Design review of the part built by this model. Coordinates are the model's own, in mm. A direction names the side the tool comes from. Coordinates: 2 decimals unless noted, no trailing zeros. Loops run counter-clockwise (first coordinate to the right, second up) from the corner with the lowest first, then second, coordinate; pieces in that order, holes last. Notation, with made-up numbers: (42.25, -35) -> (66.25, -35) arc R21 cw to (66.25, 4) -> close; hole circle Ø9 at (43.5, -30). An arc over 180 degrees is marked (long way). Answer in a Markdown table with one row per item.
```python
from build123d import *

# Parameters (mm, degrees)
F0_R     = 50.8
F1_DEPTH = 76.2
F2_DEPTH = 381
F3_R     = 25.4


with BuildPart() as f1:
    # F0 (on Front) → F1 (new body)
    with BuildSketch(Plane.XZ):
        with BuildLine():
            Line((-381, 0), (0, 0))
            Line((0, 0), (0, 508))
            ThreePointArc((0, 508), (-190.5, 698.5), (-381, 508))
            Line((-381, 508), (-381, 0))
        make_face()
        with Locations((-292.1, 127)):
            Circle(F0_R, mode=Mode.SUBTRACT)
        with Locations((-88.9, 127)):
            Circle(F0_R, mode=Mode.SUBTRACT)
        with Locations((-190.5, 508)):
            Circle(F0_R, mode=Mode.SUBTRACT)
    extrude(amount=F1_DEPTH)

    # F0 (on Front) → F2 (join)
    with BuildSketch(Plane.XZ):
        with Locations((-190.5, 508)):
            Circle(F0_R)
    extrude(amount=F2_DEPTH)

    # F3
    f3_edges = [f1.edges().sort_by_distance(p)[0] for p in [
        (-381, -38.1, 0),
        (0, -38.1, 0),
    ]]
    fillet(f3_edges, radius=F3_R)


solid = f1.part
```
(1) Tool access review of faces 1 (the cylindrical face through (-201.512, -226.466, 458.408)), 2 (the flat face through (-381, -38, 270)): name each direction out of +Z, -Z, +X, -X, +Y, -Y from which nothing blocks a thin tool from reaching the whole face with its end or side.
Evaluation:
| item | result |
|---|---|
| face 1 | -Y |
| face 2 | +Z, -Z, -X, +Y, -Y |
(2) To check wall thickness, follow probe 1 along X at (y, z) = (-24.5, 101.5); probe 2 along Z at (x, y) = (-189, -305); probe 3 along Z at (x, y) = (-292, -40). State the ranges of each line that lie inside material, in increasing order.
Evaluation:
| item | result |
|---|---|
| probe 1 | x = -381 to -336.04, -248.16 to -132.84, -44.96 to 0 |
| probe 2 | z = 457.22 to 558.78 |
| probe 3 | z = 0 to 76.2, 177.8 to 669.21 |
(3) Take a section at A-A on z = 127. Give the boundary of the cut face in (x, y).
Evaluation:
| item | result |
|---|---|
| outline | (-381, -76.2) -> (-342.9, -76.2) -> (-342.9, 0) -> (-381, 0) -> close; (-241.3, -76.2) -> (-139.7, -76.2) -> (-139.7, 0) -> (-241.3, 0) -> close; (-38.1, -76.2) -> (0, -76.2) -> (0, 0) -> (-38.1, 0) -> close |
(4) For pin 1 (6 mm diameter, centred on x = -158.5, y = -166, fed in from -Z); pin 2 (4 mm diameter, centred on x = -186.5, y = -291, fed in from +Z); pin 3 (2 mm diameter, centred on x = -71, z = 439.5, fed in from -Y), all flat-tipped, find the tip position at first contact; note any pin that passes through.
Evaluation:
| item | result |
|---|---|
| pin 1 | stops at z = 466.29 |
| pin 2 | stops at z = 558.76 |
| pin 3 | stops at y = -76.2 |
(5) Draft analysis for pull direction Z (two halves, no side actions). For faces 3 (the cylindrical face through (-245.174, -37.567, 107.543)), 4 (the flat face through (0, -38, 263)), 5 (the cylindrical face through (-373.36, -38.63, 7.24)), state which applies: pulls with the +Z half, pulls with the -Z half, needs draft (parallel to the pull), parting line crosses it, or undercut.
Evaluation:
| item | result |
|---|---|
| face 3 | undercut |
| face 4 | needs draft |
| face 5 | pulls with the -Z half |
(6) Take a section at C-C on x = -328.5. Give the boundary of the cut face in (y, z).
Evaluation:
| item | result |
|---|---|
| outline | (-76.2, 0) -> (0, 0) -> (0, 91.56) -> (-76.2, 91.56) -> close; (-76.2, 162.44) -> (0, 162.44) -> (0, 639.32) -> (-76.2, 639.32) -> close |
(7) Take a section at B-B on y = -66. Give the boundary of the cut face in (x, z).
Evaluation:
| item | result |
|---|---|
| outline | (-381, 25.4) arc R25.4 ccw to (-355.6, 0) -> (-25.4, 0) arc R25.4 ccw to (0, 25.4) -> (0, 508) arc R190.5 ccw to (-381, 508) -> close; hole circle Ø101.6 at (-292.1, 127); hole circle Ø101.6 at (-88.9, 127) |
(8) Take a section at D-D on x = -190.5. Give the boundary of the cut face in (y, z), and give its area (3 significant figures).
Evaluation:
| item | result |
|---|---|
| outline | (-381, 457.2) -> (-76.2, 457.2) -> (-76.2, 0) -> (0, 0) -> (0, 698.5) -> (-76.2, 698.5) -> (-76.2, 558.8) -> (-381, 558.8) -> close |
| area | 84,200 mm² |
